Can you work these out from the model? Positions are in its coordinate system, mm. A direction names the side the tool comes from. Round coordinates to 2 decimals unless told otherwise and drop trailing zeros. Loops run counter-clockwise (first coordinate to the right, second up) from the corner with the lowest first, then second, coordinate; pieces in that order, holes last. Notation, with made-up numbers: (-20, 20) - (-1, 20) arc R26 cw to (-1, 58) - close; hole circle Ø6 at (9, 83). An arc over 180 degrees is marked (long way). Answer as CSV lines item,"result".
Autodesk Inventor part; units mm, degrees
ref_plane "YZ Plane" through (0, 0, 0) normal (1, 0, 0) x (0, 1, 0)
ref_plane "XZ Plane" through (0, 0, 0) normal (0, 1, 0) x (-1, 0, 0)
ref_plane "XY Plane" through (0, 0, 0) normal (0, 0, 1) x (1, 0, 0)
sketch "Sketch1" plane through (0, 0, 0) normal (0, 1, 0) x (-1, 0, 0)
  point P0 (0, 0)
sketch "Sketch2" plane through (0, 0, 0) normal (0, 1, 0) x (-1, 0, 0)
  line L0 (2.7724, 24.8182) -> (-3.2276, 24.8182)
  line L1 (2.7724, 24.8182) -> (2.7724, -20.1818)
  line L2 (-3.2276, 24.8182) -> (-3.2276, -20.1818)
  line L3 (-3.2276, -20.1818) -> (-1.0276, -20.1818)
  line L4 (-1.0276, -20.1818) -> (-1.0276, -13.6818)
  line L5 (2.7724, -20.1818) -> (0.5724, -20.1818)
  line L6 (0.5724, -20.1818) -> (0.5724, -13.6818)
  arc A0 (0.5724, -13.6818) -> (-1.0276, -13.6818) centre (-0.2276, -11.8488) ccw
  point P0 (0, 0)
  dimension "d0" = 6
  dimension "d1" = 45
  dimension "d2" = 45
  dimension "d3" = 2.2
  dimension "d4" = 2.2
  dimension "d5" = 6.5
  dimension "d6" = 2
extrude "Extrusion1" add sketch "Sketch2" along normal blind 6
sketch "Sketch4" plane through (0, 0, 0) normal (0, -1, 0) x (1, 0, 0)
  line L0 (-2.7724, 24.8182) -> (3.2276, 24.8182)
  circle A0 centre (0.2276, 19.8001) radius 1.2121
  point P0 (0, 0)
extrude "Extrusion3" cut sketch "Sketch4" against normal blind 10.9375
sketch "Sketch5" plane through (3.2276, 0, 24.8182) normal (1, 0, 0) x (0, 0, -1)
  circle A0 centre (41.4031, 3) radius 1.15
  line L0 (0, 0) -> (0, 6)
  line L1 (0, 4.7) -> (22.0881, 4.7)
  line L2 (22.0881, 4.7) -> (22.0881, 1.3)
  line L3 (22.0881, 1.3) -> (0, 1.3)
  line L4 (0, 4.7) -> (0, 1.3)
  point P0 (24.8182, 0)
  dimension "d13" = 2.3
  dimension "d18" = 3.4
  dimension "d19" = 1.3
extrude "Extrusion4" cut sketch "Sketch5" against normal blind 14.6375 contours A0
extrude "Extrusion5" cut sketch "Sketch5" against normal blind 23.4625 contours L0 L1 L2 L3
properties part number "LInk1"
Q1. Imagine slicing it at D-D (y = 0.7). Write out the boundary of the cut face in (x, z).
Checks:
outline,"(-2.77, -20.18) - (-0.57, -20.18) - (-0.57, -13.68) arc R2 cw (long way) to (1.03, -13.68) - (1.03, -20.18) - (3.23, -20.18) - (3.23, 24.82) - (-2.77, 24.82) - close; hole circle Ø2.42 at (0.23, 19.8)"
Q2. We'd pull the mould along X, two halves only. Please class faces 1 (the cylindrical face through (-0.035, 0.641, 18.617)), 2 (the flat face through (2, 3, -20.182)), 3 (the flat face through (3.228, 3, -2)): pulls with the +X half, pulls with the -X half, needs draft (parallel to the pull), parting line crosses it, or undercut.
Checks:
face 1,"undercut"
face 2,"needs draft"
face 3,"pulls with the +X half"
Q3. I'm going to push a flat-ended pin straight in: pin 1 Ø1 at (x, y) = (0.5, 4) entering from +Z. Where does the tip first touch, or does it pass through?
Checks:
pin 1,"z = 2.73"
Q4. Imagine slicing it at C-C (z = -17). Write out the boundary of the cut face in (x, y).
Checks:
outline,"(-2.77, 0) - (-0.57, 0) - (-0.57, 1.93) - (-2.77, 1.93) - close; (-2.77, 4.07) - (-0.57, 4.07) - (-0.57, 6) - (-2.77, 6) - close; (1.03, 0) - (3.23, 0) - (3.23, 1.93) - (1.03, 1.93) - close; (1.03, 4.07) - (3.23, 4.07) - (3.23, 6) - (1.03, 6) - close"
Q5. Imagine slicing it at B-B (z = 5). Write out the boundary of the cut face in (x, y), then the cut area to 3 significant figures.
Checks:
outline,"(-2.77, 0) - (3.23, 0) - (3.23, 1.3) - (-2.77, 1.3) - close; (-2.77, 4.7) - (3.23, 4.7) - (3.23, 6) - (-2.77, 6) - close"
area,"15.6 mm²"
Q6. If I drill on line 1 along Y through (x, z) = (-0.25, 21.5); line 2 along X through (y, z) = (0.9, -16); line 3 along X through (y, z) = (5.5, 20.5), over which ranges is the centre line in solid material (lowest first)? Write a range as [from, to].
Checks:
line 1,"[0, 1.3], [4.7, 6]"
line 2,"[-2.77, -0.57], [1.03, 3.23]"
line 3,"[-2.77, -0.76], [1.22, 3.23]"
Q7. On a 3-axis mill with a long thin cutter (end or side, diameter ignored), from which of +Z, -Z, +X, -X, +Y, -Y can I reach the whole of each face in a straight line? I mean faces 4 (the flat face through (1.028, 2, -18)), 5 (the flat face through (0, 1.3, 14)), 6 (the flat face through (-2, 3, -20.182)). Say none if no direction works.
Checks:
face 4,"-Z, +Y, -Y"
face 5,"+Z, +X, -X"
face 6,"-Z, +X, -X, +Y, -Y"
Q8. Imagine slicing it at A-A (y = 3). Write out the boundary of the cut face in (x, z), then the cut area to 3 significant figures.
Checks:
outline,"(-2.77, -20.18) - (-0.57, -20.18) - (-0.57, -17.73) - (-2.77, -17.73) - close; (-2.77, -15.43) - (-0.57, -15.43) - (-0.57, -13.68) arc R2 cw (long way) to (1.03, -13.68) - (1.03, -15.43) - (3.23, -15.43) - (3.23, 2.73) - (-2.77, 2.73) - close; (1.03, -20.18) - (3.23, -20.18) - (3.23, -17.73) - (1.03, -17.73) - close"
area,"105 mm²"
